```python
from build123d import *

# Parameters (mm, degrees)
SKETCH023_R           = 10.75
SKETCH023_R_2         = 10.25
PAD011_DEPTH          = 250
POCKET009_DEPTH       = 3
POLARPATTERN003_COUNT = 4
CYLINDER002_R         = 5
CYLINDER002_DEPTH     = 24


with BuildPart() as part:
    # Sketch023 → Pad011 (new body)
    with BuildSketch(Plane.XY):
        Circle(SKETCH023_R)
        Circle(SKETCH023_R_2, mode=Mode.SUBTRACT)
    extrude(amount=-PAD011_DEPTH)

    # Sketch024 → Pocket009 (cut)
    with BuildSketch(Plane.XY):
        Polygon((0, 12.14), (2, 12.14), (2, 2), (12.14, 2), (12.14, 0), (0, 0), align=None)
    pocket009 = extrude(amount=-POCKET009_DEPTH, mode=Mode.SUBTRACT)

    # PolarPattern003: Pocket009 ×4 about axis
    polarpattern003_axis = Axis((0, 0, 0), (0, 0, 1))
    for i in range(1, POLARPATTERN003_COUNT):
        add(pocket009.rotate(polarpattern003_axis, i * 360 / POLARPATTERN003_COUNT), mode=Mode.SUBTRACT)

    # Cylinder002 → Cylinder002 (cut)
    with BuildSketch(Plane(origin=(0, 12, -20), x_dir=(1, 0, 0), z_dir=(0, -1, 0))):
        Circle(CYLINDER002_R)
    extrude(amount=CYLINDER002_DEPTH, mode=Mode.SUBTRACT)


with BuildPart() as part_1:
    # Body011 placement: moved
    add(part.part.moved(Location((0, 0, 4.5))))


solid = part_1.part
```
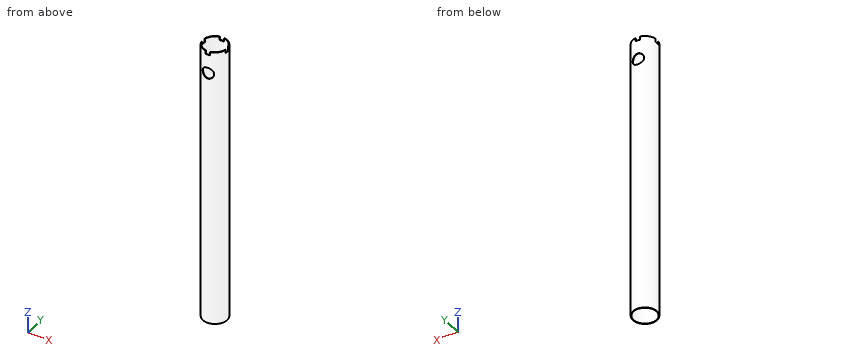
Source: CAD feature listing. Evaluate the final solid. Frame: model axes, mm. Give positions to 0.01 mm unless a question says otherwise; leave off trailing zeros. Loops run counter-clockwise (first coordinate to the right, second up) from the corner with the lowest first, then second, coordinate; pieces in that order, holes last. Notation, with made-up numbers: (78.25, 25.5) -> (122.25, 25.5) arc R29 cw to (122.25, 61.5) -> close; hole circle Ø3 at (45.25, 80). An arc over 180 degrees is marked (long way). Put each result on its own line as item: value. Start each with the question number.
1) Cut plane A-A (y = 5.75). Return loops of the section in (x, z), then the cut area to 3 significant figures.
2) Contact query for flat-ended pins moving along their axis: P1, Ø8, axis at x = 7.5, z = -63.5, coming from the -Y side; P2, Ø1.5, axis at x = -7.5, y = -1, coming from the -Z side; P3, Ø3, axis at y = -8.5, z = -96, coming from the -X side; P4, Ø6, axis at x = 7, z = -38, coming from the -Y side. Output: stop coordinate, or through.
3) Cut plane C-C (z = -194). Return loops of the section in (x, y).
4) Cut plane B-B (z = -15.5). Return loops of the section in (x, y), then the cut area to 3 significant figures.
5) Material intervals for probe 1 along Y at (x, z) = (0, -135.5); probe 2 along Y at (x, z) = (2, -135); probe 3 along X at (y, z) = (0.5, -111), sorted ascending.
Results are:
1. outline: (-9.08, -245.5) -> (-8.49, -245.5) -> (-8.49, 4.5) -> (-9.08, 4.5) -> close; (8.49, -245.5) -> (9.08, -245.5) -> (9.08, 4.5) -> (8.49, 4.5) -> close
1. area: 299 mm2
2. P1: stops at y = -10.16
2. P2: passes through
2. P3: stops at x = -8.16
2. P4: stops at y = -9.98
3. outline: circle Ø21.5 at (0, 0); hole circle Ø20.5 at (0, 0)
4. outline: (-5, -9.52) -> (-5, -8.95) arc R10.25 cw to (-5, 8.95) -> (-5, 9.52) arc R10.75 ccw to start; (5, -9.52) arc R10.75 ccw to (5, 9.52) -> (5, 8.95) arc R10.25 cw to (5, -8.95) -> close
4. area: 22.6 mm2
5. probe 1: y = -10.75 to -10.25, 10.25 to 10.75
5. probe 2: y = -10.56 to -10.05, 10.05 to 10.56
5. probe 3: x = -10.74 to -10.24, 10.24 to 10.74
